Geometry check sheet. Reference: drawing and pictorial views, mm from the part's lowest x, y, z. A direction names the side the tool comes from. Give positions to 0.01 mm unless a question says otherwise; leave off trailing zeros. Write each loop counter-clockwise with the first axis right and the second up, starting at its lowest first coordinate (ties: lowest second). Pieces come first, ordered by that corner, then holes. Notation, with made-up numbers: M -32,41.5 L -4,41.5 A21 cw -4,49.5 Z; hole C -35.5,-37 d10. An arc over 180 degrees is marked long. Write each question's results on one line, items separated by ' | '. Start each with the question number.
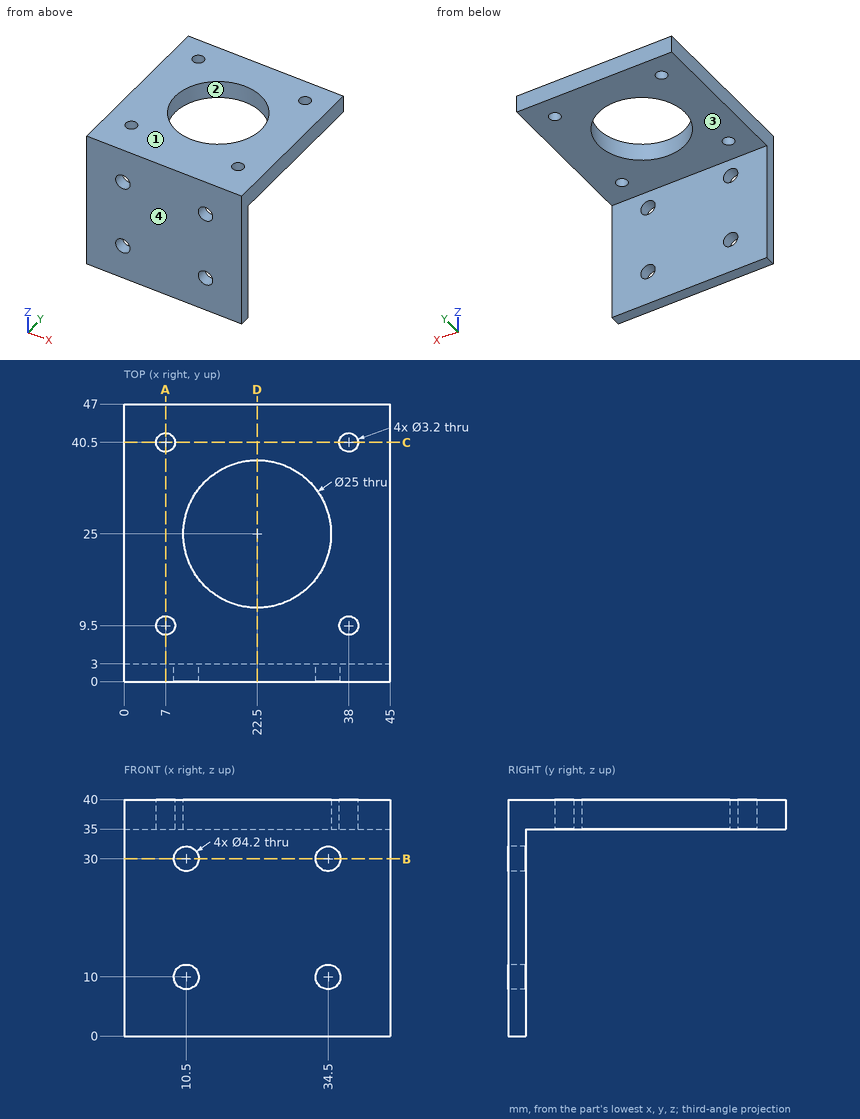
Q1. Section check B-B on z = 30. Record the boundary of the cut face in (x, y), plus the area to 3 significant figures.
Q2. Scan lines: L1, parallel to X at y = 2.3, z = 10; L2, parallel to Y at x = 38, z = 37; L3, parallel to Z at x = 8, y = 14. Record each from-to range of solid material in increasing order.
Q3. Release check for a two-part mould opening along X. For the marked faces 1 and 2 record: pulls with the +X half, pulls with the -X half, needs draft (parallel to the pull), parting line crosses it, or undercut.
Q4. Section check C-C on y = 40.5. Record the boundary of the cut face in (x, z), plus the area to 3 significant figures.
Q5. Depth check by flat-ended pin: pin 1 Ø8 at (x, y) = (28.5, 34) entering from -Z; pin 2 Ø10.5 at (x, z) = (12.5, 11.5) entering from +Y. Enter the tip coordinate at first touch or a pass-through.
Q6. Section check D-D on x = 22.5. Record the boundary of the cut face in (y, z).
Q7. Tool access check on the marked faces 3 and 4. Record the directions out of +Z, -Z, +X, -X, +Y, -Y that give a thin tool (end or side, any length) a straight path to the whole face; none if there is none.
Q8. Section check A-A on x = 7. Record the boundary of the cut face in (y, z), plus the area to 3 significant figures.
Check result:
1) outline: M 0,0 L 8.4,0 L 8.4,3 L 0,3 Z; M 12.6,0 L 32.4,0 L 32.4,3 L 12.6,3 Z; M 36.6,0 L 45,0 L 45,3 L 36.6,3 Z | area: 110 mm^2
2) L1: 0 to 8.4, 12.6 to 32.4, 36.6 to 45 | L2: 0 to 7.9, 11.1 to 38.9, 42.1 to 47 | L3: 35 to 40
3) face 1: needs draft | face 2: undercut
4) outline: M 0,35 L 5.4,35 L 5.4,40 L 0,40 Z; M 8.6,35 L 36.4,35 L 36.4,40 L 8.6,40 Z; M 39.6,35 L 45,35 L 45,40 L 39.6,40 Z | area: 193 mm^2
5) pin 1: z = 35 | pin 2: y = 3
6) outline: M 0,0 L 3,0 L 3,35 L 12.5,35 L 12.5,40 L 0,40 Z; M 37.5,35 L 47,35 L 47,40 L 37.5,40 Z
7) face 3: -Z, +X, -X, +Y | face 4: +Z, -Z, +X, -X, -Y
8) outline: M 0,0 L 3,0 L 3,35 L 7.9,35 L 7.9,40 L 0,40 Z; M 11.1,35 L 38.9,35 L 38.9,40 L 11.1,40 Z; M 42.1,35 L 47,35 L 47,40 L 42.1,40 Z | area: 308 mm^2
